from build123d import *

# Parameters (mm, degrees)
SKETCH1_W               = 270
SKETCH1_H               = 212
BOSS_EXTRUDE1_DEPTH     = 10
SKETCH2_W               = 270
SKETCH2_H               = 212
SKETCH2_W_2             = 262
SKETCH2_H_2             = 202
BOSS_EXTRUDE2_DEPTH     = 70
SKETCH3_W               = 40
SKETCH3_H               = 40
SKETCH3_W_2             = 30
SKETCH3_H_2             = 30
BOSS_EXTRUDE3_DEPTH     = 7
CHAMFER1_SIZE           = 10
SKETCH4_R               = 2.65
CUT_EXTRUDE1_DEPTH      = 207
CIRPATTERN1_COUNT       = 2
MIRROR2_COPY_1_SKETCH_R = 2.65
MIRROR2_COPY_1_DEPTH    = 207
SKETCH5_R               = 2.65
CUT_EXTRUDE2_DEPTH      = 213
FILLET1_R               = 7
SKETCH6_W               = 262
SKETCH6_H               = 202
SKETCH6_W_2             = 254
SKETCH6_H_2             = 194
BOSS_EXTRUDE4_DEPTH     = 7
SKETCH7_W               = 27
SKETCH7_H               = 13
CUT_EXTRUDE3_DEPTH      = 4
CUT_EXTRUDE4_START      = -271
SKETCH8_R               = 2.7
CUT_EXTRUDE4_DEPTH      = 272


with BuildPart() as part:
    # Sketch1 → Boss-Extrude1 (new body)
    with BuildSketch(Plane(origin=(0, 0, 0), x_dir=(1, 0, 0), z_dir=(0, 1, 0))):
        Rectangle(SKETCH1_W, SKETCH1_H)
    extrude(amount=BOSS_EXTRUDE1_DEPTH)

    # Sketch2 → Boss-Extrude2 (add)
    with BuildSketch(Plane(origin=(0, 10, 0), x_dir=(1, 0, 0), z_dir=(0, 1, 0))):
        Rectangle(SKETCH2_W, SKETCH2_H)
        Rectangle(SKETCH2_W_2, SKETCH2_H_2, mode=Mode.SUBTRACT)
    extrude(amount=BOSS_EXTRUDE2_DEPTH)

    # Sketch3 → Boss-Extrude3 (add)
    with BuildSketch(Plane(origin=(0, 10, 0), x_dir=(1, 0, 0), z_dir=(0, 1, 0))):
        Rectangle(SKETCH3_W, SKETCH3_H)
        Rectangle(SKETCH3_W_2, SKETCH3_H_2, mode=Mode.SUBTRACT)
    extrude(amount=BOSS_EXTRUDE3_DEPTH)

    # Chamfer1
    chamfer1_edges = [part.edges().sort_by_distance(p)[0] for p in [
        (0, 0, 106),
        (-135, 0, 0),
        (0, 0, -106),
        (135, 0, 0),
    ]]
    chamfer(chamfer1_edges, length=CHAMFER1_SIZE)

    # Sketch4 → Cut-Extrude1 (cut)
    with BuildSketch(Plane.XY.offset(106)):
        with Locations((83.5, 27)):
            Circle(SKETCH4_R)
        with Locations((38.5, 27)):
            Circle(SKETCH4_R)
        with Locations((61, 68)):
            Circle(SKETCH4_R)
    cut_extrude1 = extrude(amount=-CUT_EXTRUDE1_DEPTH, mode=Mode.SUBTRACT)

    # CirPattern1: Cut-Extrude1 ×2 about axis
    cirpattern1_axis = Axis((0, 84, 0), (0, -1, 0))
    for i in range(1, CIRPATTERN1_COUNT):
        add(cut_extrude1.rotate(cirpattern1_axis, i * 360 / CIRPATTERN1_COUNT), mode=Mode.SUBTRACT)

    # Mirror2: Cut-Extrude1 across plane
    add(cut_extrude1.mirror(Plane(origin=(0, 0, 0), x_dir=(0, 0, 1), z_dir=(1, 0, 0))), mode=Mode.SUBTRACT)

    # Mirror2 copy 1 sketch → Mirror2 copy 1 (cut)
    with BuildSketch(Plane(origin=(0, 0, -106), x_dir=(1, 0, 0), z_dir=(0, 0, -1))):
        with Locations((83.5, -27)):
            Circle(MIRROR2_COPY_1_SKETCH_R)
        with Locations((38.5, -27)):
            Circle(MIRROR2_COPY_1_SKETCH_R)
        with Locations((61, -68)):
            Circle(MIRROR2_COPY_1_SKETCH_R)
    extrude(amount=-MIRROR2_COPY_1_DEPTH, mode=Mode.SUBTRACT)

    # Sketch5 → Cut-Extrude2 (cut, through all)
    with BuildSketch(Plane.XY.offset(106)):
        with Locations((-120, 70)):
            Circle(SKETCH5_R)
        with Locations((-120, 30)):
            Circle(SKETCH5_R)
        with Locations((-100, 40)):
            Circle(SKETCH5_R)
    cut_extrude2 = extrude(amount=-CUT_EXTRUDE2_DEPTH, mode=Mode.SUBTRACT)

    # Mirror1: Cut-Extrude2 across plane
    add(cut_extrude2.mirror(Plane(origin=(0, 0, 0), x_dir=(0, 0, 1), z_dir=(1, 0, 0))), mode=Mode.SUBTRACT)

    # Fillet1
    fillet1_edges = [part.edges().sort_by_distance(p)[0] for p in [
        (125, 0, 0),
        (0, 0, 96),
        (-125, 0, 0),
        (0, 0, -96),
    ]]
    fillet(fillet1_edges, radius=FILLET1_R)

    # Sketch6 → Boss-Extrude4 (add)
    with BuildSketch(Plane(origin=(0, 10, 0), x_dir=(1, 0, 0), z_dir=(0, 1, 0))):
        Rectangle(SKETCH6_W, SKETCH6_H)
        Rectangle(SKETCH6_W_2, SKETCH6_H_2, mode=Mode.SUBTRACT)
    extrude(amount=BOSS_EXTRUDE4_DEPTH)

    # Sketch7 → Cut-Extrude3 (cut)
    with BuildSketch(Plane(origin=(135, 0, 0), x_dir=(0, 0, -1), z_dir=(1, 0, 0))):
        with Locations((0, 69.5)):
            Rectangle(SKETCH7_W, SKETCH7_H)
    extrude(amount=-CUT_EXTRUDE3_DEPTH, mode=Mode.SUBTRACT)

    # Sketch8 → Cut-Extrude4 (cut)
    with BuildSketch(Plane.ZY.offset(135).offset(CUT_EXTRUDE4_START)):
        with Locations((-92, 68)):
            Circle(SKETCH8_R)
    cut_extrude4 = extrude(amount=CUT_EXTRUDE4_DEPTH, mode=Mode.SUBTRACT)

    # Mirror3: Cut-Extrude4 across plane
    add(cut_extrude4.mirror(Plane.XY), mode=Mode.SUBTRACT)


solid = part.part
The model under review builds one solid part; all positions refer to its coordinate system, in mm. A direction names the side the tool comes from. Give positions to 0.01 mm unless a question says otherwise; leave off trailing zeros. Write each loop counter-clockwise with the first axis right and the second up, starting at its lowest first coordinate (ties: lowest second). Pieces come first, ordered by that corner, then holes. Notation, with made-up numbers: M -30,59.25 L 13,59.25 A34 cw 13,94.25 Z; hole C 38.25,30 d3. An arc over 180 degrees is marked long. One line per question, with ' | ' between items. Start each with the question number.
Item 1: For faces 1 (the flat face through (-1, 80, -103)), 2 (the flat face through (131, 48, 1)), list the 3-axis set-ups (+Z, -Z, +X, -X, +Y, -Y) from which the entire face can be reached by the end or side of a thin tool; tool diameter is ignored.
Item 2: Wall thickness on line 1 (Z direction, x = -122.5, y = 67); line 2 (X direction, y = 13.5, z = 54.5); line 3 (X direction, y = 55, z = -50.5): over which ranges is each line inside the solid? List them lowest first. Write a range as from..to.
Item 3: Draft analysis for pull direction Z (two halves, no side actions). For faces 3 (the flat face through (-2, 45, -106)), 4 (the flat face through (-131, 48, 1)), 5 (the cylindrical face through (-81.397, 25.388, -103.535)), state which applies: released by +Z, released by -Z, zero draft, split by the parting line, or undercut.
Item 4: For pin 1 (3 mm diameter, centred on x = -0.5, z = 74, fed in from +Y); pin 2 (5 mm diameter, centred on y = 68, z = -92, fed in from -X), all flat-tipped, find the tip position at first contact; note any pin that passes through.
Item 5: We need section A-A on x = 30.5. Write out the cut boundary in (y, z).
Item 6: We need section B-B on y = 54. Write out the cut boundary in (x, z).
Item 7: We need section C-C on z = -30. Write out the cut boundary in (x, y), plus the area to 3 significant figures.
Results found:
1) face 1: +Z, -Z, +X, -X, +Y | face 2: +Y
2) line 1: z = -106..-101, 101..106 | line 2: x = -135..-127, 127..135 | line 3: x = -135..-131, 131..135
3) face 3: released by -Z | face 4: undercut | face 5: zero draft
4) pin 1: stops at y = 10 | pin 2: passes through
5) outline: M 0,-93.1 A7 ccw 2.05,-98.05 L 10,-106 L 80,-106 L 80,-101 L 17,-101 L 17,-97 L 10,-97 L 10,97 L 17,97 L 17,101 L 80,101 L 80,106 L 10,106 L 2.05,98.05 A7 ccw 0,93.1 Z
6) outline: M -135,-106 L 135,-106 L 135,106 L -135,106 Z; hole M -131,-101 L 131,-101 L 131,101 L -131,101 Z
7) outline: M -135,10 L -127.05,2.05 A7 ccw -122.1,0 L 122.1,0 A7 ccw 127.05,2.05 L 135,10 L 135,80 L 131,80 L 131,17 L 127,17 L 127,10 L -127,10 L -127,17 L -131,17 L -131,80 L -135,80 Z | area: 3,210 mm2
